Read the model definition and answer for the solid it produces. Units are mm, in the model's axes. Give positions to 0.01 mm unless a question says otherwise; leave off trailing zeros. Write each loop counter-clockwise with the first axis right and the second up, starting at its lowest first coordinate (ties: lowest second). Pieces come first, ordered by that corner, then holes. Notation, with made-up numbers: M 13.25,-5 L 37.25,-5 A21 ccw 37.25,32 Z; hole C 1.5,30 d7. An arc over 180 degrees is marked long. Use a Markdown table: item, result. Add a question column.
Item 1: A cutting plane is placed at C-C on y = 1.5. Determine the outline of the cut face in (x, z).
Item 2: A cutting plane is placed at A-A on x = 29. Determine the outline of the cut face in (y, z).
Item 3: A cutting plane is placed at D-D on y = -32. Determine the outline of the cut face in (x, z).
Item 4: A cutting plane is placed at B-B on z = 1.45. Determine the outline of the cut face in (x, y).
Item 5: Given P1, Ø1, axis at x = 39, z = 2, coming from the +Y side; P2, Ø1, axis at x = 33, z = 0.5, coming from the +Y side; P3, Ø7, axis at x = 30.76, y = 30.76, coming from the +Z side, each flat-ended and moving along its own axis, determine where each tip first touches the part or whether it passes through.
Item 6: Consider probe 1 along Y at (x, z) = (21, 1.8); probe 2 along Y at (x, z) = (13, 1.6); probe 3 along Y at (x, z) = (28, 0.65). Determine where each line is inside the solid, lowest interval first. Write a range as [from, to].
from build123d import *

# Parameters (mm, degrees)
F2_DEPTH = 3
F0_R     = 3.75
F3_DEPTH = 25
F5_DEPTH = 25


with BuildPart() as f2:
    # F1 (on Top) → F2 (new body)
    with BuildSketch(Plane.XY):
        with BuildLine():
            Line((15.300233, 43.614948), (6.077594, 23.609497))
            ThreePointArc((6.077594, 23.609497), (6.020288, 20.390579), (8.353267, 18.172037))
            ThreePointArc((8.353267, 18.172037), (20, 0), (8.353267, -18.172037))
            ThreePointArc((8.353267, -18.172037), (6.020288, -20.390579), (6.077594, -23.609497))
            Line((6.077594, -23.609497), (15.300233, -43.614948))
            ThreePointArc((15.300233, -43.614948), (17.707769, -45.748102), (20.907488, -45.418905))
            ThreePointArc((20.907488, -45.418905), (50, 0), (20.907488, 45.418905))
            ThreePointArc((20.907488, 45.418905), (17.707769, 45.748102), (15.300233, 43.614948))
        make_face()
    extrude(amount=F2_DEPTH)

    # F0 (on Top) → F3 (cut)
    with BuildSketch(Plane.XY):
        with Locations((30.759145, 30.759145)):
            Circle(F0_R)
        with Locations((30.759145, -30.759145)):
            Circle(F0_R)
    extrude(amount=F3_DEPTH, mode=Mode.SUBTRACT)

    # F4 (on face) → F5 (cut)
    with BuildSketch(Plane.XY.offset(3)):
        with BuildLine():
            ThreePointArc((16.917114, 25.402395), (12.757267, 24.568324), (13.591338, 20.408477))
            ThreePointArc((13.591338, 20.408477), (24.52, 0), (13.591338, -20.408477))
            ThreePointArc((13.591338, -20.408477), (12.757267, -24.568324), (16.917114, -25.402395))
            ThreePointArc((16.917114, -25.402395), (30.52, 0), (16.917114, 25.402395))
        make_face()
    extrude(amount=-F5_DEPTH, mode=Mode.SUBTRACT)


solid = f2.part
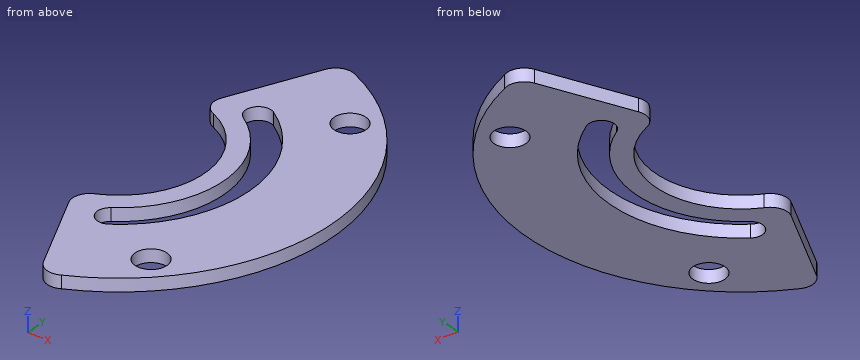
Filled in:
| question | item | result |
|---|---|---|
| 1 | outline | M 19.94,0 L 24.47,0 L 24.47,3 L 19.94,3 Z; M 30.48,0 L 49.98,0 L 49.98,3 L 30.48,3 Z |
| 2 | outline | M -40.73,0 L -34.07,0 L -34.07,3 L -40.73,3 Z; M -27.45,0 L -9.51,0 L -9.51,3 L -27.45,3 Z; M 9.51,0 L 27.45,0 L 27.45,3 L 9.51,3 Z; M 34.07,0 L 40.73,0 L 40.73,3 L 34.07,3 Z |
| 3 | outline | M 9.95,0 L 27.22,0 L 27.22,3 L 9.95,3 Z; M 34.3,0 L 38.42,0 L 38.42,3 L 34.3,3 Z |
| 4 | outline | M 6.08,-23.61 L 15.3,-43.61 A4 ccw 20.91,-45.42 A50 ccw 20.91,45.42 A4 ccw 15.3,43.61 L 6.08,23.61 A4 ccw 8.35,18.17 A20 cw 8.35,-18.17 A4 ccw Z; hole M 13.59,-20.41 A3 ccw 16.92,-25.4 A30.52 ccw 16.92,25.4 A3 ccw 13.59,20.41 A24.52 cw Z; hole C 30.76,-30.76 d7.5; hole C 30.76,30.76 d7.5 |
| 5 | P1 | y = 31.9 |
| 5 | P2 | y = 38 |
| 5 | P3 | through |
| 6 | probe 1 | [-45.38, -22.15], [-12.66, 12.66], [22.15, 45.38] |
| 6 | probe 2 | [-38.63, -24.88], [-20.93, -15.2], [15.2, 20.93], [24.88, 38.63] |
| 6 | probe 3 | [-41.42, -33.3], [-28.22, -12.14], [12.14, 28.22], [33.3, 41.42] |
